from build123d import *

# Parameters (mm, degrees)
F0_R     = 2.5
F1_DEPTH = 4


# Not quite as in the source:
# - a pattern or mirror of a feature is missing from the dataset's text; its kind, count and spacing are read off the source's solid


with BuildPart() as f1:
    # F0 (on Front) → F1 (new body)
    with BuildSketch(Plane.XZ):
        with BuildLine():
            Line((30, 35), (-30, 35))
            ThreePointArc((-30, 35), (-33.5355339059, 33.5355339059), (-35, 30))
            Line((-35, 30), (-35, -30))
            ThreePointArc((-35, -30), (-33.5355339059, -33.5355339059), (-30, -35))
            Line((-30, -35), (30, -35))
            ThreePointArc((30, -35), (33.5355339059, -33.5355339059), (35, -30))
            Line((35, -30), (35, 30))
            ThreePointArc((35, 30), (33.5355339059, 33.5355339059), (30, 35))
        make_face()
        with Locations((-25, -25)):
            Circle(F0_R, mode=Mode.SUBTRACT)
        with Locations((25, -25)):
            Circle(F0_R, mode=Mode.SUBTRACT)
        with Locations((-25, 25)):
            Circle(F0_R, mode=Mode.SUBTRACT)
        with Locations((25, 25)):
            Circle(F0_R, mode=Mode.SUBTRACT)
    extrude(amount=F1_DEPTH)

    # F1_copies: F1 across plane


with BuildPart() as f1_1:
    add(f1.part)
    add(f1.part.mirror(Plane(origin=(0, -4, 0), x_dir=(0, 0, -1), z_dir=(0, -1, 0))))


solid = f1_1.part
The model under review builds one solid part; all positions refer to its coordinate system, in mm. Round coordinates to 2 decimals unless told otherwise and drop trailing zeros. Write each loop counter-clockwise with the first axis right and the second up, starting at its lowest first coordinate (ties: lowest second). Pieces come first, ordered by that corner, then holes. Notation, with made-up numbers: (55.25, 65) -> (96.25, 65) arc R32 ccw to (96.25, 101) -> close; hole circle Ø4 at (5.5, 10.25). An arc over 180 degrees is marked (long way). Answer as a JSON object with one key per item and string values.
1. We need section C-C on y = -1. State the section outline as (x, z) points.
Results found:
{"outline": "(-35, -30) arc R5 ccw to (-30, -35) -> (30, -35) arc R5 ccw to (35, -30) -> (35, 30) arc R5 ccw to (30, 35) -> (-30, 35) arc R5 ccw to (-35, 30) -> close; hole circle Ø5 at (-25, -25); hole circle Ø5 at (-25, 25); hole circle Ø5 at (25, -25); hole circle Ø5 at (25, 25)"}
2. We need section B-B on x = -25. State the section outline as (y, z) points.
Results found:
{"outline": "(-8, -35) -> (0, -35) -> (0, -27.5) -> (-8, -27.5) -> close; (-8, -22.5) -> (0, -22.5) -> (0, 22.5) -> (-8, 22.5) -> close; (-8, 27.5) -> (0, 27.5) -> (0, 35) -> (-8, 35) -> close"}
3. We need section A-A on z = -25. State the section outline as (x, y) points.
Results found:
{"outline": "(-35, -8) -> (-27.5, -8) -> (-27.5, 0) -> (-35, 0) -> close; (-22.5, -8) -> (22.5, -8) -> (22.5, 0) -> (-22.5, 0) -> close; (27.5, -8) -> (35, -8) -> (35, 0) -> (27.5, 0) -> close"}
4. To check wall thickness, follow line 1 along Z through (x, y) = (-25, -2.25); line 2 along Z through (x, y) = (-24.5, -7.25); line 3 along X through (y, z) = (-4.5, -23). State the ranges of each line that lie inside material, in increasing order.
Results found:
{"line 1": "z = -35 to -27.5, -22.5 to 22.5, 27.5 to 35", "line 2": "z = -35 to -27.45, -22.55 to 22.55, 27.45 to 35", "line 3": "x = -35 to -26.5, -23.5 to 23.5, 26.5 to 35"}
5. The part is to be moulded in two halves that separate along Z. For faces 1 (the face through (33, -4, -34)), 2 (the face through (0, -8, 0)), 3 (the face through (24.67, -4.06, 27.48)), say which applies: pulls with the +Z half, pulls with the -Z half, needs draft (parallel to the pull), parting line crosses it, or undercut.
Results found:
{"face 1": "pulls with the -Z half", "face 2": "needs draft", "face 3": "undercut"}
